The model under review builds one solid part; all positions refer to its coordinate system, in mm. A direction names the side the tool comes from. Give positions to 0.01 mm unless a question says otherwise; leave off trailing zeros. Order: outer loops, then holes, each group sorted by start corner. A loop starts at its lowest first (then second) coordinate and runs counter-clockwise, first axis right, second up. Notation, with made-up numbers: (0.5, 9.5) - (19.5, 9.5) arc R22 cw to (19.5, 32.5) - close; hole circle Ø6 at (16, 71). An arc over 180 degrees is marked (long way). Use CSV: the item, a comma, the result in double quotes.
```python
from build123d import *

# Parameters (mm, degrees)
SKETCH1_W           = 127
SKETCH1_H           = 78.74
BOSS_EXTRUDE1_DEPTH = 19.05
SKETCH2_W           = 50.8
SKETCH2_H           = 78.74
BOSS_EXTRUDE2_DEPTH = 19.05
SKETCH3_W           = 127
SKETCH3_H           = 78.74
BOSS_EXTRUDE3_DEPTH = 19.05
CHAMFER1_SIZE       = 10.16


with BuildPart() as part:
    # Sketch1 → Boss-Extrude1 (new body)
    with BuildSketch(Plane.XY):
        Rectangle(SKETCH1_W, SKETCH1_H)
    extrude(amount=BOSS_EXTRUDE1_DEPTH)

    # Sketch2 → Boss-Extrude2 (add)
    with BuildSketch(Plane.XY.offset(19.05)):
        with Locations((-38.1, 0)):
            Rectangle(SKETCH2_W, SKETCH2_H)
        with Locations((38.1, 0)):
            Rectangle(SKETCH2_W, SKETCH2_H)
    extrude(amount=BOSS_EXTRUDE2_DEPTH)

    # Sketch3 → Boss-Extrude3 (add)
    with BuildSketch(Plane.XY.offset(38.1)):
        Rectangle(SKETCH3_W, SKETCH3_H)
    extrude(amount=BOSS_EXTRUDE3_DEPTH)

    # Chamfer1
    chamfer1_edges = [part.edges().sort_by_distance(p)[0] for p in [
        (-63.5, 0, 57.15),
        (0, -39.37, 57.15),
        (63.5, 0, 57.15),
        (0, 39.37, 57.15),
        (0, -39.37, 0),
        (-63.5, 0, 0),
        (0, 39.37, 0),
        (63.5, 0, 0),
        (63.5, -39.37, 28.575),
        (-63.5, -39.37, 28.575),
        (-63.5, 39.37, 28.575),
        (63.5, 39.37, 28.575),
    ]]
    chamfer(chamfer1_edges, length=CHAMFER1_SIZE)


solid = part.part
```
Item 1: Take a section at C-C, the plane x = -4. Give the boundary of the cut face in (y, z), and give its area (3 significant figures).
Results list:
outline,"(-39.37, 10.16) - (-29.21, 0) - (29.21, 0) - (39.37, 10.16) - (39.37, 19.05) - (-39.37, 19.05) - close; (-39.37, 38.1) - (39.37, 38.1) - (39.37, 46.99) - (29.21, 57.15) - (-29.21, 57.15) - (-39.37, 46.99) - close"
area,"2,790 mm2"
Item 2: Take a section at D-D, the plane z = 5. Give the boundary of the cut face in (x, y), and give its area (3 significant figures).
Results list:
outline,"(-58.34, -29.21) - (-53.34, -34.21) - (53.34, -34.21) - (58.34, -29.21) - (58.34, 29.21) - (53.34, 34.21) - (-53.34, 34.21) - (-58.34, 29.21) - close"
area,"7,930 mm2"
Item 3: Mouldability with a two-part tool opening along Z and no side actions: class faces 3 (the face through (57.2, -32.3, 50.2)), 4 (the face through (-56.41, 33.09, 6.95)), 5 (the face through (-12.7, -1, 28)) as pulls with the +Z half, pulls with the -Z half, needs draft (parallel to the pull), parting line crosses it, or undercut.
Results list:
face 3,"pulls with the +Z half"
face 4,"pulls with the -Z half"
face 5,"undercut"
Item 4: Take a section at B-B, the plane y = -33. Give the boundary of the cut face in (x, z).
Results list:
outline,"(-59.71, 10.16) - (-53.34, 3.79) - (53.34, 3.79) - (59.71, 10.16) - (59.71, 46.99) - (53.34, 53.36) - (-53.34, 53.36) - (-59.71, 46.99) - close; hole (-12.7, 19.05) - (12.7, 19.05) - (12.7, 38.1) - (-12.7, 38.1) - close"
Item 5: Wall thickness on L1, parallel to X at y = -28.5, z = 36.5; L2, parallel to Z at x = 1.5, y = 22; L3, parallel to X at y = 23, z = 10: over which ranges is each line inside the solid? List them lowest first.
Results list:
L1,"x = -63.5 to -12.7, 12.7 to 63.5"
L2,"z = 0 to 19.05, 38.1 to 57.15"
L3,"x = -63.34 to 63.34"
Item 6: Take a section at A-A, the plane z = 32. Give the boundary of the cut face in (x, y), and give its area (3 significant figures).
Results list:
outline,"(-63.5, -29.21) - (-53.34, -39.37) - (-12.7, -39.37) - (-12.7, 39.37) - (-53.34, 39.37) - (-63.5, 29.21) - close; (12.7, -39.37) - (53.34, -39.37) - (63.5, -29.21) - (63.5, 29.21) - (53.34, 39.37) - (12.7, 39.37) - close"
area,"7,790 mm2"
Item 7: Tool access review of faces 1 (the face through (0, 1, 38.1)), 2 (the face through (-56.4, -33.1, 50.2)): name each direction out of +Z, -Z, +X, -X, +Y, -Y from which nothing blocks a thin tool from reaching the whole face with its end or side.
Results list:
face 1,"+Y, -Y"
face 2,"+Z, -X, -Y"
Item 8: Clearance check with a flat-ended pin moving along its axis: pin 1 (2 mm diameter, centred on y = 30.5, z = 49.5, fed in from -X). State where the tip first meets the part, or that it passes through.
Results list:
pin 1,"stops at x = -61.11"
